Part model, mm, in its own coordinate system. A direction names the side the tool comes from. Give positions to 0.01 mm unless a question says otherwise; leave off trailing zeros. Write each loop counter-clockwise with the first axis right and the second up, starting at its lowest first coordinate (ties: lowest second). Pieces come first, ordered by that corner, then holes.
```python
from build123d import *

# Parameters (mm, degrees)
SKETCH_W     = 15.5
SKETCH_H     = 10
PAD_DEPTH    = 2
SKETCH001_R  = 1.235
PAD001_DEPTH = 2.8
FILLET_R     = 2.5
FILLET001_R  = 1
SKETCH002_W  = 4
SKETCH002_H  = 10
PAD002_DEPTH = 0.25


with BuildPart() as part:
    # Sketch → Pad (new body)
    with BuildSketch(Plane.XY):
        Rectangle(SKETCH_W, SKETCH_H)
    extrude(amount=PAD_DEPTH)

    # Sketch001 (on Face5 of Pad) → Pad001 (join)
    with BuildSketch(Plane(origin=(0, 0, 0), x_dir=(1, 0, 0), z_dir=(0, 0, -1))):
        with Locations((-4, 0)):
            Circle(SKETCH001_R)
        with Locations((4, 0)):
            Circle(SKETCH001_R)
    extrude(amount=PAD001_DEPTH)

    # Fillet
    fillet_edges = [part.edges().sort_by_distance(p)[0] for p in [
        (7.75, 5, 1),
        (7.75, -5, 1),
        (-7.75, -5, 1),
        (-7.75, 5, 1),
    ]]
    fillet(fillet_edges, radius=FILLET_R)

    # Fillet001
    fillet001_edges = [part.edges().sort_by_distance(p)[0] for p in [
        (0, -5, 2),
        (7.75, 0, 2),
        (0, 5, 2),
        (-7.75, 0, 2),
    ]]
    fillet(fillet001_edges, radius=FILLET001_R)

    # Sketch002 (on Face4 of Fillet001) → Pad002 (join)
    with BuildSketch(Plane(origin=(0, 0, 0), x_dir=(1, 0, 0), z_dir=(0, 0, -1))):
        Rectangle(SKETCH002_W, SKETCH002_H)
    extrude(amount=PAD002_DEPTH)


solid = part.part
```
1) Saw through at D-D, the plane y = 0. Write the cut outline in (x, z) (3 decimals), then the cut area to 3 significant figures.
Answers follow:
outline: (-7.75, 0) - (-5.235, 0) - (-5.235, -2.8) - (-2.765, -2.8) - (-2.765, 0) - (-2, 0) - (-2, -0.25) - (2, -0.25) - (2, 0) - (2.765, 0) - (2.765, -2.8) - (5.235, -2.8) - (5.235, 0) - (7.75, 0) - (7.75, 1) arc R1 ccw to (6.75, 2) - (-6.75, 2) arc R1 ccw to (-7.75, 1) - close
area: 45.4 mm2
2) 3-axis set-ups, long thin cutter, end or side, ignore diameter. For faces 5 (the face through (6.998, 4.287, 0.507)), 6 (the face through (-2.86, 0.47, -1.38)): which of +Z, -Z, +X, -X, +Y, -Y reach the whole face in a straight line?
Answers follow:
face 5: +Z, -Z, +X, +Y
face 6: -Z
3) Saw through at A-A, the plane y = 2. Write the cut outline in (x, z).
Answers follow:
outline: (-7.75, 0) - (-2, 0) - (-2, -0.25) - (2, -0.25) - (2, 0) - (7.75, 0) - (7.75, 1) arc R1 ccw to (6.75, 2) - (-6.75, 2) arc R1 ccw to (-7.75, 1) - close
4) Saw through at B-B, the plane z = -0.7. Write the cut outline in (x, y) (3 decimals), then the cut area to 3 significant figures.
Answers follow:
outline: circle Ø2.47 at (-4, 0); circle Ø2.47 at (4, 0)
area: 9.58 mm2
5) Two-plate mould, pull along X, no slides. Class faces 1 (the face through (6.998, -4.287, 0.507)), 2 (the face through (0, 0, -0.25)), 3 (the face through (-7.037, -4.248, 0.507)), 4 (the face through (-0.1, 5, 0.5)): +X half, -X half, draft (parallel to the pull), parting line (faces both ways), or undercut.
Answers follow:
face 1: +X half
face 2: undercut
face 3: -X half
face 4: draft
6) Wall check: L1, parallel to X at y = 3.75, z = -0.15; L2, parallel to X at y = 0.75, z = -0.65; L3, parallel to Z at x = -6.5, y = -1. Give the ranges that are in metal, low to high.
Answers follow:
L1: x = -2 to 2
L2: x = -4.98 to -3.02, 3.02 to 4.98
L3: z = 0 to 2
7) Saw through at C-C, the plane x = 4. Write the cut outline in (y, z) (3 decimals).
Answers follow:
outline: (-5, 0) - (-1.235, 0) - (-1.235, -2.8) - (1.235, -2.8) - (1.235, 0) - (5, 0) - (5, 1) arc R1 ccw to (4, 2) - (-4, 2) arc R1 ccw to (-5, 1) - close
8) Pin check, flat tips, straight feed: pin 1 Ø1.5 at (y, z) = (0.5, -2.5) entering from +X (3 decimals); pin 2 Ø2 at (x, y) = (0.5, 2) entering from -Z. Stop position of each tip, or through.
Answers follow:
pin 1: stops at x = 5.235
pin 2: stops at z = -0.25
